from build123d import *

# Parameters (mm, degrees)
SKETCH2_R           = 12.7
BOSS_EXTRUDE1_DEPTH = 6.35
FILLET1_R           = 0.635


with BuildPart() as part:
    # Sketch1 → Revolve1 (revolve)
    with BuildSketch(Plane.XY):
        with BuildLine():
            ThreePointArc((0, -12.7), (-12.7, 0), (0, 12.7))
            Line((0, 12.7), (0, -12.7))
        make_face()
        with BuildLine():
            ThreePointArc((-4.7625, 11.773215098), (-2.425919233, 12.466150804), (0, 12.7))
            Line((0, 12.7), (0, 38.1))
            Line((0, 38.1), (-4.7625, 38.1))
            Line((-4.7625, 38.1), (-4.7625, 11.773215098))
        make_face()
    revolve(axis=Axis((0, 12.7, 0), (0, 1, 0)))

    # Sketch2 → Boss-Extrude1 (add, symmetric)
    with BuildSketch(Plane(origin=(0, 0, 0), x_dir=(0, 0, -1), z_dir=(1, 0, 0))):
        with Locations((0, 38.1)):
            Circle(SKETCH2_R)
    extrude(amount=BOSS_EXTRUDE1_DEPTH, both=True)

    # Fillet1
    fillet1_edges = [part.edges().sort_by_distance(p)[0] for p in [
        (4.762500002, 25.4, -1e-09),
        (-6.35, 38.1, 12.7),
        (6.35, 38.1, 12.7),
        (4.7625, 11.773215098, 0),
    ]]
    fillet(fillet1_edges, radius=FILLET1_R)

    # Sketch4 → CBORE for 1/4 Pan Head Machine Screw1 (revolve, cut)
    with BuildSketch(Plane(origin=(6.35, 38.1, 0), x_dir=(0, 0, -1), z_dir=(0, 1, 0))):
        Polygon((0, 0), (0, 19.05), (3.3782, 19.05), (3.3782, 4.445), (6.74624, 4.445), (6.74624, 0.635), (7.38124, 0), align=None)
    revolve(axis=Axis((12.7, 38.1, 0), (-1, 0, 0)), mode=Mode.SUBTRACT)


solid = part.part
Geometry: final body of the model. Coordinates: model frame, mm. A direction names the side the tool comes from. Give positions to 0.01 mm unless a question says otherwise; leave off trailing zeros. Write each loop counter-clockwise with the first axis right and the second up, starting at its lowest first coordinate (ties: lowest second). Pieces come first, ordered by that corner, then holes. Notation, with made-up numbers: (-6.75, 32) - (41.25, 32) arc R16 ccw to (41.25, 45) - close; hole circle Ø3 at (86, -0.75). An arc over 180 degrees is marked (long way). Return JSON: item names as keys, results as strings. Group by question number.
1) Line query: line 1 (Y direction, x = 3.95, z = 0); line 2 (Y direction, x = -4, z = 0); line 3 (Z direction, x = 6, y = 38.5). Output: solid intervals per line, ascending.
2) Section A-A on y = 38.1. Return the cut outline in (x, z) (3 decimals).
3) First-contact query: P1, Ø1, axis at x = -7.5, z = -6, coming from the +Y side; P2, Ø5, axis at y = 39.5, z = -7.5, coming from the +X side; P3, Ø1.5, axis at x = -6.5, z = -9, coming from the +Y side. Flat tips, straight axial feed; report the tip coordinate or a pass-through.
4) Section C-C on x = 9.25. Return the cut outline in (y, z).
5) Section B-B on y = 19.5. Return the cut outline in (x, z) (1 decimal).
6) Mould query, pull axis Y, two halves, no side actions, for faces 4 (the flat face through (6.35, 33, 6)), 5 (the cylindrical face through (-2.16, 34.75, 0.44)). Classes: released by +Y, released by -Y, zero draft, split by the parting line, or undercut.
7) Set-up query: faces 1 (the cylindrical face through (3.837, 44.686, 1.462)), 2 (the cylindrical face through (4.758, 18.954, 0.209)), 3 (the flat face through (-6.35, 36, -3)). Return all of +Z, -Z, +X, -X, +Y, -Y with unobstructed straight access to the full face (end or side cutting, diameter ignored); none if empty.
Filled in:
{
 "1": {"line 1": "y = -12.07 to 31.35, 44.85 to 50.8", "line 2": "y = -12.05 to 34.72, 41.48 to 50.8", "line 3": "z = -12.63 to -7.02, 7.02 to 12.63"},
 "2": {"outline": "(-6.35, -12.065) arc R0.635 ccw to (-5.715, -12.7) - (5.715, -12.7) arc R0.635 ccw to (6.35, -12.065) - (6.35, -7.381) - (5.715, -6.746) - (1.905, -6.746) - (1.905, -3.378) - (-6.35, -3.378) - close; (-6.35, 3.378) - (1.905, 3.378) - (1.905, 6.746) - (5.715, 6.746) - (6.35, 7.381) - (6.35, 12.065) arc R0.635 ccw to (5.715, 12.7) - (-5.715, 12.7) arc R0.635 ccw to (-6.35, 12.065) - close"},
 "3": {"P1": "stops at y = 8.85", "P2": "stops at x = 6.35", "P3": "stops at y = 47.5"},
 "4": {"outline": "circle Ø17.4 at (0, 0)"},
 "5": {"outline": "circle Ø9.5 at (0, 0)"},
 "6": {"face 4": "zero draft", "face 5": "undercut"},
 "7": {"face 1": "+X", "face 2": "none", "face 3": "+Z, -Z, -X, +Y"}
}
